Autodesk Inventor part; units mm, degrees
ref_plane "YZ Plane" through (0, 0, 0) normal (1, 0, 0) x (0, 1, 0)
ref_plane "XZ Plane" through (0, 0, 0) normal (0, 1, 0) x (-1, 0, 0)
ref_plane "XY Plane" through (0, 0, 0) normal (0, 0, 1) x (1, 0, 0)
sketch "Sketch1" plane through (0, 0, 0) normal (0, 1, 0) x (-1, 0, 0)
  line L0 (0, 0) -> (0, -218)
  arc A0 (0, 0) -> (-9, 0) centre (-4.5, 0) ccw
  line L1 (-9, 0) -> (-13.5, 0)
  line L2 (4.5, 0) -> (4.5, -218)
  arc A1 (4.5, 0) -> (-13.5, 0) centre (-4.5, 0) ccw
  line L3 (0, 0) -> (-17, 0) construction
  line L4 (52, -109) -> (-119, -109) construction
  line L5 (0, -218) -> (0, 0)
  arc A2 (-9, -218) -> (0, -218) centre (-4.5, -218) ccw
  line L6 (-9, -218) -> (-13.5, -218)
  line L7 (4.5, -218) -> (4.5, 0)
  arc A3 (-13.5, -218) -> (4.5, -218) centre (-4.5, -218) ccw
  point P0 (4.5, -109)
  dimension "d0" = 218
  dimension "d1" = 9
  dimension "d2" = 4.5
  dimension "d3" = 218
  dimension "d4" = 4.5
  dimension "d5" = 9
  dimension "d6" = 4.5
  dimension "d7" = 18
extrude "Extrusion1" add sketch "Sketch1" along normal blind 23
sketch "Sketch2" plane through (0, 0, 0) normal (1, 0, 0) x (0, 0, -1)
  circle A0 centre (109, 11.5) radius 2.5
  line L0 (0, 23) -> (218, 23)
  line L1 (0, 0) -> (0, 23)
  line L2 (33.5, 4) -> (43.5, 4) construction
  line L3 (43.5, 4) -> (43.5, 19) construction
  line L4 (43.5, 19) -> (33.5, 19) construction
  line L5 (33.5, 19) -> (33.5, 4) construction
  line L6 (33.5, 4) -> (43.5, 19) construction
  line L7 (43.5, 4) -> (33.5, 19) construction
  circle A1 centre (43.5, 19) radius 2
  circle A2 centre (33.5, 19) radius 2
  circle A3 centre (33.5, 4) radius 2
  circle A4 centre (43.5, 4) radius 2
  line L8 (0, 0) -> (218, 0)
  line L9 (21.5, 5.5) -> (21.5, 17.5) construction
  circle A5 centre (21.5, 17.5) radius 1.5
  circle A6 centre (21.5, 5.5) radius 1.5
  line L10 (109, 37.5143) -> (109, -14.5143) construction
  line L11 (184.5, 4) -> (174.5, 4) construction
  line L12 (174.5, 4) -> (174.5, 19) construction
  line L13 (174.5, 19) -> (184.5, 19) construction
  line L14 (184.5, 19) -> (184.5, 4) construction
  line L15 (184.5, 4) -> (174.5, 19) construction
  line L16 (174.5, 4) -> (184.5, 19) construction
  circle A7 centre (174.5, 19) radius 2
  circle A8 centre (184.5, 19) radius 2
  circle A9 centre (184.5, 4) radius 2
  circle A10 centre (174.5, 4) radius 2
  line L17 (196.5, 5.5) -> (196.5, 17.5) construction
  circle A11 centre (196.5, 17.5) radius 1.5
  circle A12 centre (196.5, 5.5) radius 1.5
  point P0 (38.5, 11.5)
  point P1 (179.5, 11.5)
  dimension "d10" = 5
  dimension "d11" = 11.5
  dimension "d12" = 109
  dimension "d13" = 4
  dimension "d14" = 4
  dimension "d15" = 4
  dimension "d16" = 4
  dimension "d17" = 4
  dimension "d18" = 4
  dimension "d19" = 65.5
  dimension "d20" = 10
  dimension "d21" = 3
  dimension "d22" = 3
  dimension "d23" = 5.5
  dimension "d24" = 5.5
  dimension "d25" = 12
hole "Hole1" at (0, 17.5, -21.5) at (0, 5.5, -21.5) at (0, 17.5, -196.5) at (0, 5.5, -196.5) direction (-1, 0, 0) diameter 3 end through all
hole "Hole2" at (0, 19, -184.5) at (0, 19, -174.5) at (0, 4, -184.5) at (0, 4, -174.5) at (0, 19, -33.5) at (0, 19, -43.5) at (0, 4, -33.5) at (0, 4, -43.5) direction (-1, 0, 0) diameter 4 end through all
hole "Hole3" at (0, 11.5, -109) direction (-1, 0, 0) diameter 5 end through all
properties part number "HUDSON-1-07 FRONT BUFFERR BEAM"
The model under review builds one solid part; all positions refer to its coordinate system, in mm. A direction names the side the tool comes from. Round coordinates to 2 decimals unless told otherwise and drop trailing zeros. Loops run counter-clockwise (first coordinate to the right, second up) from the corner with the lowest first, then second, coordinate; pieces in that order, holes last. Notation, with made-up numbers: (-3, 8.25) - (34, 8.25) arc R21 ccw to (34, 38.25) - close; hole circle Ø4 at (80.5, -24.5). An arc over 180 degrees is marked (long way). Write each question's results on one line, items separated by ' | '. Start each with the question number.
Q1. Draft analysis for pull direction Y (two halves, no side actions). For faces 4 (the cylindrical face through (-2.282, 17.017, -43.24)), 5 (the flat face through (-1, 23, -108)), 6 (the cylindrical face through (-2.282, 18.912, -182.502)), 7 (the cylindrical face through (4.6, 11.3, 4.5)), state which applies: pulls with the +Y half, pulls with the -Y half, needs draft (parallel to the pull), parting line crosses it, or undercut.
Q2. Take a section at C-C on y = 11.5. Give the boundary of the cut face in (x, z).
Q3. Tool access review of faces 1 (the cylindrical face through (-2.282, 10.749, -111.385)), 2 (the cylindrical face through (4.4, 11.3, -222.5)), 3 (the flat face through (11, 11, -218)): name each direction out of +Z, -Z, +X, -X, +Y, -Y from which nothing blocks a thin tool from reaching the whole face with its end or side.
Q4. Take a section at D-D on z = -33.5. Give the boundary of the cut face in (x, y), plus the area to 3 significant figures.
Q5. Wall thickness on line 1 along Y through (x, z) = (-3.3, -196.5); line 2 along Z through (x, y) = (-2, 20.25); line 3 along X through (y, z) = (22.25, -179.5): over which ranges is each line inside the solid? List them lowest first. Write a range as [from, to].
Q6. Take a section at B-B on x = 4.5. Give the boundary of the cut face in (y, z), plus the area to 3 significant figures.
Q7. Insertion check: P1, Ø5, axis at x = 3.5, z = -88.5, coming from the -Y side; P2, Ø3, axis at y = 5, z = -189, coming from the +X side; P3, Ø3.5, axis at x = 12, y = 13.5, coming from the -Z side; P4, Ø4, axis at x = 1.5, y = 17, coming from the -Z side. Each pin has a flat end and moves straight along its axis. Give the tip position at first contact, or say it passes through.
Q8. Take a section at A-A on z = -109. Give the boundary of the cut face in (x, y).
Data:
1) face 4: undercut | face 5: pulls with the +Y half | face 6: undercut | face 7: needs draft
2) outline: (-4.5, -218) arc R9 ccw to (13.5, -218) - (9, -218) arc R4.5 cw to (0, -218) - (0, -111.5) - (-4.5, -111.5) - close; (-4.5, -106.5) - (0, -106.5) - (0, 0) arc R4.5 cw to (9, 0) - (13.5, 0) arc R9 ccw to (-4.5, 0) - close
3) face 1: +X, -X | face 2: +Y, -Y | face 3: +X, +Y, -Y
4) outline: (-4.5, 0) - (0, 0) - (0, 2) - (-4.5, 2) - close; (-4.5, 6) - (0, 6) - (0, 17) - (-4.5, 17) - close; (-4.5, 21) - (0, 21) - (0, 23) - (-4.5, 23) - close | area: 67.5 mm²
5) line 1: y = [0, 4], [7, 16], [19, 23] | line 2: z = [-224.22, -186.06], [-182.94, -176.06], [-172.94, -45.06], [-41.94, -35.06], [-31.94, 6.22] | line 3: x = [-4.5, 0]
6) outline: (0, -227) - (23, -227) - (23, -222.5) - (0, -222.5) - close; (0, 4.5) - (23, 4.5) - (23, 9) - (0, 9) - close | area: 207 mm²
7) P1: passes through | P2: stops at x = 0 | P3: stops at z = -224.92 | P4: stops at z = -226.94
8) outline: (-4.5, 0) - (0, 0) - (0, 9) - (-4.5, 9) - close; (-4.5, 14) - (0, 14) - (0, 23) - (-4.5, 23) - close
